For this review, take the finished solid that the model builds, in its own axes (mm). Coordinates: 2 decimals unless noted, no trailing zeros. Order: outer loops, then holes, each group sorted by start corner. A loop starts at its lowest first (then second) coordinate and runs counter-clockwise, first axis right, second up. Notation, with made-up numbers: (-24.75, 24.25) - (10.25, 24.25) arc R16 cw to (10.25, 49.25) - close; hole circle Ø4 at (-0.75, -7.75). An arc over 180 degrees is marked (long way). One line per item, written item: value. Start each with the question number.
(1) Consider section A-A on y = 42.5. Write out the cut boundary in (x, z), then the cut area to 3 significant figures.
(2) Consider section B-B on y = 16. Write out the cut boundary in (x, z), then the cut area to 3 significant figures.
(3) Consider section D-D on y = 50. Write out the cut boundary in (x, z).
(4) Consider section C-C on z = -0.5. Count the separate pieces of the cut face and the enclosed holes in it, then the cut area to 3 significant figures.
(5) Mouldability with a two-part tool opening along X and no side actions: class faces 1 (the cylindrical face through (-3.905, 26.622, -0.867)), 2 (the cylindrical face through (3.07, 49.62, 1.19)), 3 (the cylindrical face through (-2.44, 43.86, 0.54)) as released by +X, released by -X, zero draft, split by the parting line, or undercut.
(6) To check wall thickness, follow line 1 along Y through (x, z) = (3.05, 0); line 2 along X through (y, z) = (43.75, 0); line 3 along Y through (x, z) = (2.5, -1). State the ranges of each line that lie inside material, in increasing order.
(7) Clearance check with flat-ended pins moving along their axes: pin 1 (1.5 mm diameter, centred on x = -0.5, z = -2, fed in from +Y); pin 2 (1 mm diameter, centred on x = 1, z = -1, fed in from +Y); pin 3 (2 mm diameter, centred on y = 16, z = 0, fed in from -X). State where each tip first meets the part, or that it passes through.
```python
from build123d import *

# Parameters (mm, degrees)
SKETCH1_R                   = 4
BOSS_EXTRUDE1_DEPTH         = 54
F_5_0MM_DOWEL_HOLE2_D       = 5
F_5_0MM_DOWEL_HOLE2_DEPTH   = 20
F_5_0MM_DOWEL_HOLE2_TIP     = 1.502151548
SKETCH14_W                  = 1.25
SKETCH14_H                  = 4
TAP_DRILL_FOR_M3X0_5_TAP4_D = 2.5


with BuildPart() as part:
    # Sketch1 → Boss-Extrude1 (new body)
    with BuildSketch(Plane(origin=(0, 0, 0), x_dir=(1, 0, 0), z_dir=(0, 1, 0))):
        with Locations(Location((0, 0, 0), (0, 0, 270))):
            Circle(SKETCH1_R)
    extrude(amount=BOSS_EXTRUDE1_DEPTH)

    # Ø5.0mm Dowel Hole2
    with Locations(Plane.ZX.offset(54)):
        with Locations((0, 0)):
            Hole(F_5_0MM_DOWEL_HOLE2_D / 2, depth=F_5_0MM_DOWEL_HOLE2_DEPTH)
            with Locations((0, 0, -(F_5_0MM_DOWEL_HOLE2_DEPTH + F_5_0MM_DOWEL_HOLE2_TIP / 2))):  # 118° drill point
                Cone(0, F_5_0MM_DOWEL_HOLE2_D / 2, F_5_0MM_DOWEL_HOLE2_TIP, mode=Mode.SUBTRACT)

    # Sketch12 → Tap Drill for M3x0.5 Tap2 (revolve, cut)
    with BuildSketch(Plane.ZX.offset(50)):
        Polygon((0, 0), (0, 20.751075774), (1.25, 20), (1.25, 0), align=None)
    revolve(axis=Axis((-6.35, 50, 0), (1, 0, 0)), mode=Mode.SUBTRACT)

    # Sketch14 → Tap Drill for M3x0.5 Tap3 (revolve, cut)
    with BuildSketch(Plane.ZX.offset(16)):
        with Locations((0.625, 2)):
            Rectangle(SKETCH14_W, SKETCH14_H)
    revolve(axis=Axis((-6.35, 16, 0), (1, 0, 0)), mode=Mode.SUBTRACT)

    # Tap Drill for M3x0.5 Tap4 (through all)
    with Locations(Plane(origin=(0, 0, 0), x_dir=(0, 0, -1), z_dir=(1, 0, 0))):
        with Locations((0, 16)):
            Hole(TAP_DRILL_FOR_M3X0_5_TAP4_D / 2)


solid = part.part
```
Geometry check:
1. outline: circle Ø8 at (0, 0); hole circle Ø5 at (0, 0)
1. area: 30.6 mm^2
2. outline: (-3.8, -1.25) arc R4 ccw to (3.8, -1.25) - close; (-3.8, 1.25) - (3.8, 1.25) arc R4 ccw to start
2. area: 30.6 mm^2
3. outline: (2.17, -1.25) arc R2.5 cw (long way) to (2.17, 1.25) - (3.8, 1.25) arc R4 ccw (long way) to (3.8, -1.25) - close
4. separate pieces: 3
4. enclosed holes: 0
4. area: 306 mm^2
5. face 1: split by the parting line
5. face 2: zero draft
5. face 3: undercut
6. line 1: y = 0 to 14.75, 17.25 to 48.75, 51.25 to 54
6. line 2: x = -4 to -2.5, 2.5 to 4
6. line 3: y = 0 to 15.25, 16.75 to 49.25, 50.75 to 54
7. pin 1: stops at y = 54
7. pin 2: stops at y = 33.65
7. pin 3: passes through
